from build123d import *

# Parameters (mm, degrees)
F3_W = 76.2
F3_H = 3.2


with BuildPart() as f1:
    # F0 (on Top) → F1 (revolve)
    with BuildSketch(Plane.XY):
        Polygon((44.843938002, 15.85), (57.15, 15.85), (57.15, 19.05), (44.45, 19.05), (19.05, 12.7), (-19.05, 12.7), (-57.15, 25.4), (-69.85, 25.4), (-69.85, 22.2), (-57.6692885125, 22.2), (-19.5692885125, 9.5), (19.443938002, 9.5), align=None)
    revolve(axis=Axis((-6.35, 0, 0), (1, 0, 0)))

    # F3 (on offset) → F4 (join, up to the next surface of F1)
    with BuildSketch(Plane.XZ.offset(30.48)):
        Rectangle(F3_W, F3_H)
    extrude(until=Until.NEXT, dir=(0, 1, 0))


solid = f1.part
CAD build for the part. Positions are in the model's coordinates, mm. A direction names the side the tool comes from. Give positions to 0.01 mm unless a question says otherwise; leave off trailing zeros. Order: outer loops, then holes, each group sorted by start corner. A loop starts at its lowest first (then second) coordinate and runs counter-clockwise, first axis right, second up. Notation, with made-up numbers: (71.25, 6.5) - (117.25, 6.5) arc R10 ccw to (117.25, 24.5) - close; hole circle Ø6 at (-25, 32). An arc over 180 degrees is marked (long way). Write each question's results on one line, items separated by ' | '.
1. Pin check, flat tips, straight feed: pin 1 (5 mm diameter, centred on y = 2, z = -5, fed in from -X); pin 2 (1.6 mm diameter, centred on y = -27, z = 0.5, fed in from -X); pin 3 (19.5 mm diameter, centred on x = 16, y = -22.5, fed in from +Z); pin 4 (5 mm diameter, centred on x = 36.5, z = 16, fed in from +Y). Stop position of each tip, or through.
Calculated:
pin 1: passes through | pin 2: stops at x = -38.1 | pin 3: stops at z = 1.6 | pin 4: stops at y = 10.59
2. Saw through at B-B on x = -15.5. List the corners of the cut face in (y, z), and give its area (3 significant figures).
Calculated:
outline: (-30.48, -1.6) - (-12.6, -1.6) arc R12.7 ccw (long way) to (-12.6, 1.6) - (-30.48, 1.6) - close; hole circle Ø19 at (0, 0) | area: 280 mm2
3. Probe L1, parallel to Z at x = 53, y = 0; L2, parallel to Z at x = 1, y = 0; L3, parallel to Z at x = 10.5, y = -19. List the from-to ranges inside material, lowest first. Write a range as from..to.
Calculated:
L1: z = -19.05..-15.85, 15.85..19.05 | L2: z = -12.7..-9.5, 9.5..12.7 | L3: z = -1.6..1.6
4. Saw through at C-C on x = -61. List the corners of the cut face in (y, z).
Calculated:
outline: circle Ø50.8 at (0, 0); hole circle Ø44.4 at (0, 0)
5. Saw through at D-D on x = -44. List the corners of the cut face in (y, z).
Calculated:
outline: circle Ø42.03 at (0, 0); hole circle Ø35.29 at (0, 0)
6. 3-axis set-ups, long thin cutter, end or side, ignore diameter. For faces 1 (the face through (-38.1, -25, 0)), 2 (the face through (-1, -22, 1.6)), 3 (the face through (28.75, 14.427, 4.543)), 4 (the face through (-63.67, 11.93, 18.72)): which of +Z, -Z, +X, -X, +Y, -Y reach the whole face in a straight line?
Calculated:
face 1: +Z, -Z, -Y | face 2: +Z, -Y | face 3: none | face 4: -X
7. Pull direction Z, two halves, no side cores. Call faces 5 (the face through (50.71, -15.12, -11.59)), 6 (the face through (-1, -30.48, 0)), 7 (the face through (-34.119, 13.687, 4.31)), 8 (the face through (51.08, 15.12, 4.76)): released by +Z, released by -Z, zero draft, split by the parting line, or undercut.
Calculated:
face 5: split by the parting line | face 6: zero draft | face 7: undercut | face 8: undercut
8. Saw through at A-A on y = 0. List the corners of the cut face in (x, z), and give its area (3 significant figures).
Calculated:
outline: (-69.85, -25.4) - (-57.15, -25.4) - (-19.05, -12.7) - (19.05, -12.7) - (44.45, -19.05) - (57.15, -19.05) - (57.15, -15.85) - (44.84, -15.85) - (19.44, -9.5) - (-19.57, -9.5) - (-57.67, -22.2) - (-69.85, -22.2) - close; (-69.85, 22.2) - (-57.67, 22.2) - (-19.57, 9.5) - (19.44, 9.5) - (44.84, 15.85) - (57.15, 15.85) - (57.15, 19.05) - (44.45, 19.05) - (19.05, 12.7) - (-19.05, 12.7) - (-57.15, 25.4) - (-69.85, 25.4) - close | area: 831 mm2
